Read the model definition and answer for the solid it produces. Units are mm, in the model's axes. A direction names the side the tool comes from. Give positions to 0.01 mm unless a question says otherwise; leave off trailing zeros. Loops run counter-clockwise (first coordinate to the right, second up) from the corner with the lowest first, then second, coordinate; pieces in that order, holes last. Notation, with made-up numbers: (63, 67) -> (115, 67) arc R19 ccw to (115, 86) -> close; hole circle Ø7 at (58.25, -22). An arc over 180 degrees is marked (long way). Return JSON: item names as keys, results as strings. Group by question number.
from build123d import *

# Parameters (mm, degrees)
BOSS_EXTRUDE1_DEPTH     = 1.5
CUT_EXTRUDE1_DEPTH      = 52.061237744
CUT_EXTRUDE1_DEPTH_BACK = 52.061237744
SKETCH2_W               = 24
SKETCH2_H               = 24
FILLET1_R               = 5
M2X0_4_TAPPED_HOLE1_D   = 1.6
F_1_5MM_DOWEL_HOLE1_D   = 1.5


with BuildPart() as part:
    # Sketch1 → Boss-Extrude1 (new, symmetric)
    with BuildSketch(Plane(origin=(0, 0, 0), x_dir=(1, 0, 0), z_dir=(0, 1, 0))):
        Polygon((0, 0), (34.748434417, 0), (42, 14.5), (34.748434417, 29), (0, 29), align=None)
    extrude(amount=BOSS_EXTRUDE1_DEPTH, both=True)

    # Sketch2 → Cut-Extrude1 (cut, two sides: drawn at the far end of the back side and taken through both)
    with BuildSketch(Plane(origin=(0, 0, 0), x_dir=(1, 0, 0), z_dir=(0, 1, 0)).offset(-CUT_EXTRUDE1_DEPTH_BACK)):
        with Locations((15, 14.5)):
            Rectangle(SKETCH2_W, SKETCH2_H)
    extrude(amount=CUT_EXTRUDE1_DEPTH + CUT_EXTRUDE1_DEPTH_BACK, mode=Mode.SUBTRACT)

    # Fillet1
    fillet1_edges = [part.edges().sort_by_distance(p)[0] for p in [
        (3, 0, -2.5),
        (3, 0, -26.5),
        (27, 0, -26.5),
        (27, 0, -2.5),
    ]]
    fillet(fillet1_edges, radius=FILLET1_R)

    # M2x0.4 Tapped Hole1 (through all)
    with Locations(Plane(origin=(1.5, 1.5, -27), x_dir=(0, 0, 1), z_dir=(0, 1, 0))):
        with Locations((0, 0), (0, 27), (9.25, 36.248434417), (15.75, 36.248434417), (23, 27), (23, 0)):
            Hole(M2X0_4_TAPPED_HOLE1_D / 2)

    # Ø1.5mm Dowel Hole1 (through all)
    with Locations(Plane(origin=(32.5, 1.5, -16), x_dir=(0, 0, 1), z_dir=(0, 1, 0))):
        with Locations((0, 0), (10, 0)):
            Hole(F_1_5MM_DOWEL_HOLE1_D / 2)


solid = part.part
1. Which of the six approach directions +Z, -Z, +X, -X, +Y, -Y give full straight-line access (tool end or side, diameter ignored) to faces 5 (the flat face through (18, 0, -29)), 6 (the flat face through (27, 0, -14))?
2. Section C-C on z = -4 is taken. Determine the outline of the cut face in (x, y).
3. Flat-ended cylindrical pins translate along their axes: pin 1 Ø1 at (x, z) = (37.75, -17.75) entering from -Y; pin 2 Ø1 at (y, z) = (0, -4.5) entering from +X. Find the tip coordinate at first contact, or state that the pin passes through.
4. Determine the mould class of faces 1 (the flat face through (38.3, 0, -7.1)), 2 (the flat face through (3, 0, -14)), 3 (the flat face through (0, 0, -15)), 4 (the flat face through (17, 0, 0)) for opening direction X: pulls with the +X half, pulls with the -X half, needs draft (parallel to the pull), parting line crosses it, or undercut.
5. Straight lines are drawn through the part: line 1 (Z direction, x = 32.5, y = 0.2); line 2 (Z direction, x = 19.5, y = 0.3); line 3 (Z direction, x = 28, y = -0.6). For each, find the intervals that lie inside material, in ascending order. Write a range as from..to.
6. Section D-D on y = -0.7 is taken. State how many separate pieces and enclosed holes the cut face has, then the cut area to 3 significant figures.
7. Section A-A on x = 28.5 is taken. Determine the outline of the cut face in (y, z), then the cut area to 3 significant figures.
8. Section B-B on x = 19 is taken. Determine the outline of the cut face in (y, z).
Completed:
{
 "1": {"face 5": "-Z, +X, -X, +Y, -Y", "face 6": "+Y, -Y"},
 "2": {"outline": "(0, -1.5) -> (0.7, -1.5) -> (0.7, 1.5) -> (0, 1.5) -> close; (2.3, -1.5) -> (4.43, -1.5) -> (4.43, 1.5) -> (2.3, 1.5) -> close; (25.57, -1.5) -> (27.7, -1.5) -> (27.7, 1.5) -> (25.57, 1.5) -> close; (29.3, -1.5) -> (36.75, -1.5) -> (36.75, 1.5) -> (29.3, 1.5) -> close"},
 "3": {"pin 1": "passes through", "pin 2": "stops at x = 37.25"},
 "4": {"face 1": "pulls with the +X half", "face 2": "undercut", "face 3": "pulls with the -X half", "face 4": "needs draft"},
 "5": {"line 1": "z = -29..-16.75, -15.25..-6.75, -5.25..0", "line 2": "z = -29..-26.5, -2.5..0", "line 3": "z = -29..-27.62, -26.38..-4.62, -3.38..0"},
 "6": {"separate pieces": "1", "enclosed holes": "9", "area": "543 mm²"},
 "7": {"outline": "(-1.5, -29) -> (1.5, -29) -> (1.5, -27.8) -> (-1.5, -27.8) -> close; (-1.5, -26.2) -> (1.5, -26.2) -> (1.5, -4.8) -> (-1.5, -4.8) -> close; (-1.5, -3.2) -> (1.5, -3.2) -> (1.5, 0) -> (-1.5, 0) -> close", "area": "77.4 mm²"},
 "8": {"outline": "(-1.5, -29) -> (1.5, -29) -> (1.5, -26.5) -> (-1.5, -26.5) -> close; (-1.5, -2.5) -> (1.5, -2.5) -> (1.5, 0) -> (-1.5, 0) -> close"}
}
